```python
from build123d import *

# Parameters (mm, degrees)
SKETCH1_W           = 619.76
SKETCH1_H           = 314.96
SKETCH1_W_2         = 609.6
SKETCH1_H_2         = 304.8
EXTRUDE_THIN1_DEPTH = 152.4
SKETCH2_W           = 873.76
SKETCH2_H           = 568.96
SKETCH2_W_2         = 619.76
SKETCH2_H_2         = 314.96
BOSS_EXTRUDE1_DEPTH = 5.08
SKETCH3_W           = 619.76
SKETCH3_H           = 314.96
BOSS_EXTRUDE2_DEPTH = 2.54
SKETCH4_R           = 4.445
CUT_EXTRUDE1_DEPTH  = 155.94


with BuildPart() as part:
    # Sketch1 → Extrude-Thin1 (new body)
    with BuildSketch(Plane(origin=(0, 0, 0), x_dir=(1, 0, 0), z_dir=(0, 1, 0))):
        Rectangle(SKETCH1_W, SKETCH1_H)
        Rectangle(SKETCH1_W_2, SKETCH1_H_2, mode=Mode.SUBTRACT)
    extrude(amount=-EXTRUDE_THIN1_DEPTH)

    # Sketch2 → Boss-Extrude1 (add)
    with BuildSketch(Plane(origin=(0, 0, 0), x_dir=(1, 0, 0), z_dir=(0, 1, 0))):
        Rectangle(SKETCH2_W, SKETCH2_H)
        Rectangle(SKETCH2_W_2, SKETCH2_H_2, mode=Mode.SUBTRACT)
    extrude(amount=-BOSS_EXTRUDE1_DEPTH)

    # Sketch3 → Boss-Extrude2 (add)
    with BuildSketch(Plane.XZ.offset(152.4)):
        Rectangle(SKETCH3_W, SKETCH3_H)
    extrude(amount=BOSS_EXTRUDE2_DEPTH)

    # Sketch4 → Cut-Extrude1 (cut, through all)
    with BuildSketch(Plane(origin=(0, 0, 0), x_dir=(1, 0, 0), z_dir=(0, 1, 0))):
        with Locations((-398.78, 246.38)):
            Circle(SKETCH4_R)
        with Locations((-342.9, 246.38)):
            Circle(SKETCH4_R)
        with Locations((-342.9, 190.5)):
            Circle(SKETCH4_R)
        with Locations((-398.78, 190.5)):
            Circle(SKETCH4_R)
        with Locations((-266.7, 246.38)):
            Circle(SKETCH4_R)
        with Locations((-266.7, 190.5)):
            Circle(SKETCH4_R)
        with Locations((-210.82, 190.5)):
            Circle(SKETCH4_R)
        with Locations((-210.82, 246.38)):
            Circle(SKETCH4_R)
        with Locations((-210.82, -190.5)):
            Circle(SKETCH4_R)
        with Locations((-210.82, -246.38)):
            Circle(SKETCH4_R)
        with Locations((-266.7, -246.38)):
            Circle(SKETCH4_R)
        with Locations((-266.7, -190.5)):
            Circle(SKETCH4_R)
        with Locations((-398.78, -190.5)):
            Circle(SKETCH4_R)
        with Locations((-342.9, -190.5)):
            Circle(SKETCH4_R)
        with Locations((-342.9, -246.38)):
            Circle(SKETCH4_R)
        with Locations((-398.78, -246.38)):
            Circle(SKETCH4_R)
        with Locations((210.82, -246.38)):
            Circle(SKETCH4_R)
        with Locations((210.82, -190.5)):
            Circle(SKETCH4_R)
        with Locations((266.7, -190.5)):
            Circle(SKETCH4_R)
        with Locations((266.7, -246.38)):
            Circle(SKETCH4_R)
        with Locations((398.78, -246.38)):
            Circle(SKETCH4_R)
        with Locations((342.9, -246.38)):
            Circle(SKETCH4_R)
        with Locations((342.9, -190.5)):
            Circle(SKETCH4_R)
        with Locations((398.78, -190.5)):
            Circle(SKETCH4_R)
        with Locations((398.78, 190.5)):
            Circle(SKETCH4_R)
        with Locations((342.9, 190.5)):
            Circle(SKETCH4_R)
        with Locations((266.7, 190.5)):
            Circle(SKETCH4_R)
        with Locations((210.82, 190.5)):
            Circle(SKETCH4_R)
        with Locations((210.82, 246.38)):
            Circle(SKETCH4_R)
        with Locations((266.7, 246.38)):
            Circle(SKETCH4_R)
        with Locations((342.9, 246.38)):
            Circle(SKETCH4_R)
        with Locations((398.78, 246.38)):
            Circle(SKETCH4_R)
        with Locations((0, 271.78)):
            Circle(SKETCH4_R)
        with Locations((0, 170.18)):
            Circle(SKETCH4_R)
        with Locations((-424.18, 0)):
            Circle(SKETCH4_R)
        with Locations((-322.58, 0)):
            Circle(SKETCH4_R)
        with Locations((0, -271.78)):
            Circle(SKETCH4_R)
        with Locations((0, -170.18)):
            Circle(SKETCH4_R)
        with Locations((424.18, 0)):
            Circle(SKETCH4_R)
        with Locations((322.58, 0)):
            Circle(SKETCH4_R)
    extrude(amount=-CUT_EXTRUDE1_DEPTH, mode=Mode.SUBTRACT)


solid = part.part
```
Geometry: final body of the model. Coordinates: model frame, mm. A direction names the side the tool comes from. Round coordinates to 2 decimals unless told otherwise and drop trailing zeros. Write each loop counter-clockwise with the first axis right and the second up, starting at its lowest first coordinate (ties: lowest second). Pieces come first, ordered by that corner, then holes.
Item 1: Section query A-A (x = -127.5). Return loops of the section in (y, z), plus the area to 3 significant figures.
Item 2: Pin query (flat end, axial travel): P1, Ø8, axis at x = 266.7, z = -246.38, coming from the -Y side; P2, Ø12, axis at x = -218.5, z = 59, coming from the +Y side; P3, Ø1, axis at x = 143.5, y = -113, coming from the +Z side; P4, Ø1, axis at y = -76.5, z = 71.5, coming from the -X side. Return the tip coordinate at first contact, or that it passes through.
Item 3: Section query C-C (z = -84.5). Return loops of the section in (x, y), plus the area to 3 significant figures.
Item 4: Material intervals for L1, parallel to Z at x = 210.82, y = -1.5 (3 decimals); L2, parallel to Z at x = -398, y = -2; L3, parallel to Z at x = -210, y = -1, sorted ascending.
Item 5: Section query B-B (y = -21.5). Return loops of the section in (x, z), plus the area to 3 significant figures.
Item 6: Set-up query: faces 1 (the face through (-4, -79, -157.48)), 2 (the face through (-309.88, -79, -2)), 3 (the face through (-4, -154.94, 2)), 4 (the face through (-4, -75, -152.4)), 5 (the face through (-6, 0, -194)). Return all of +Z, -Z, +X, -X, +Y, -Y with unobstructed straight access to the full face (end or side cutting, diameter ignored); none if empty.
Item 7: Section query D-D (z = 225). Return loops of the section in (x, y), plus the area to 3 significant figures.
Item 8: Mould query, pull axis Z, two halves, no side actions, for faces 6 (the face through (-4, -152.4, 2)), 7 (the face through (309.88, -79, -2)), 8 (the face through (-4, -79, 157.48)). Classes: +Z half, -Z half, draft (parallel to the pull), parting line (faces both ways), or undercut.
Completed:
1. outline: (-154.94, -157.48) - (-5.08, -157.48) - (-5.08, -284.48) - (0, -284.48) - (0, -152.4) - (-152.4, -152.4) - (-152.4, 152.4) - (0, 152.4) - (0, 284.48) - (-5.08, 284.48) - (-5.08, 157.48) - (-154.94, 157.48) - close
1. area: 3,640 mm2
2. P1: passes through
2. P2: stops at y = -152.4
2. P3: stops at z = 157.48
2. P4: stops at x = -309.88
3. outline: (-436.88, -5.08) - (-309.88, -5.08) - (-309.88, -154.94) - (309.88, -154.94) - (309.88, -5.08) - (436.88, -5.08) - (436.88, 0) - (304.8, 0) - (304.8, -152.4) - (-304.8, -152.4) - (-304.8, 0) - (-436.88, 0) - close
3. area: 4,410 mm2
4. L1: z = -284.48 to -250.825, -241.935 to -194.945, -186.055 to -152.4, 152.4 to 186.055, 194.945 to 241.935, 250.825 to 284.48
4. L2: z = -284.48 to -250.76, -242 to -194.88, -186.12 to 186.12, 194.88 to 242, 250.76 to 284.48
4. L3: z = -284.48 to -250.75, -242.01 to -194.87, -186.13 to -152.4, 152.4 to 186.13, 194.87 to 242.01, 250.75 to 284.48
5. outline: (-309.88, -157.48) - (309.88, -157.48) - (309.88, 157.48) - (-309.88, 157.48) - close; hole (-304.8, -152.4) - (304.8, -152.4) - (304.8, 152.4) - (-304.8, 152.4) - close
5. area: 9,390 mm2
6. face 1: -Z, +X, -X, -Y
6. face 2: +Z, -Z, -X, -Y
6. face 3: +Z, -Z, +X, -X, -Y
6. face 4: +Y
6. face 5: +Z, -Z, +X, -X, +Y
7. outline: (-436.88, -5.08) - (436.88, -5.08) - (436.88, 0) - (-436.88, 0) - close
7. area: 4,440 mm2
8. face 6: undercut
8. face 7: draft
8. face 8: +Z half
